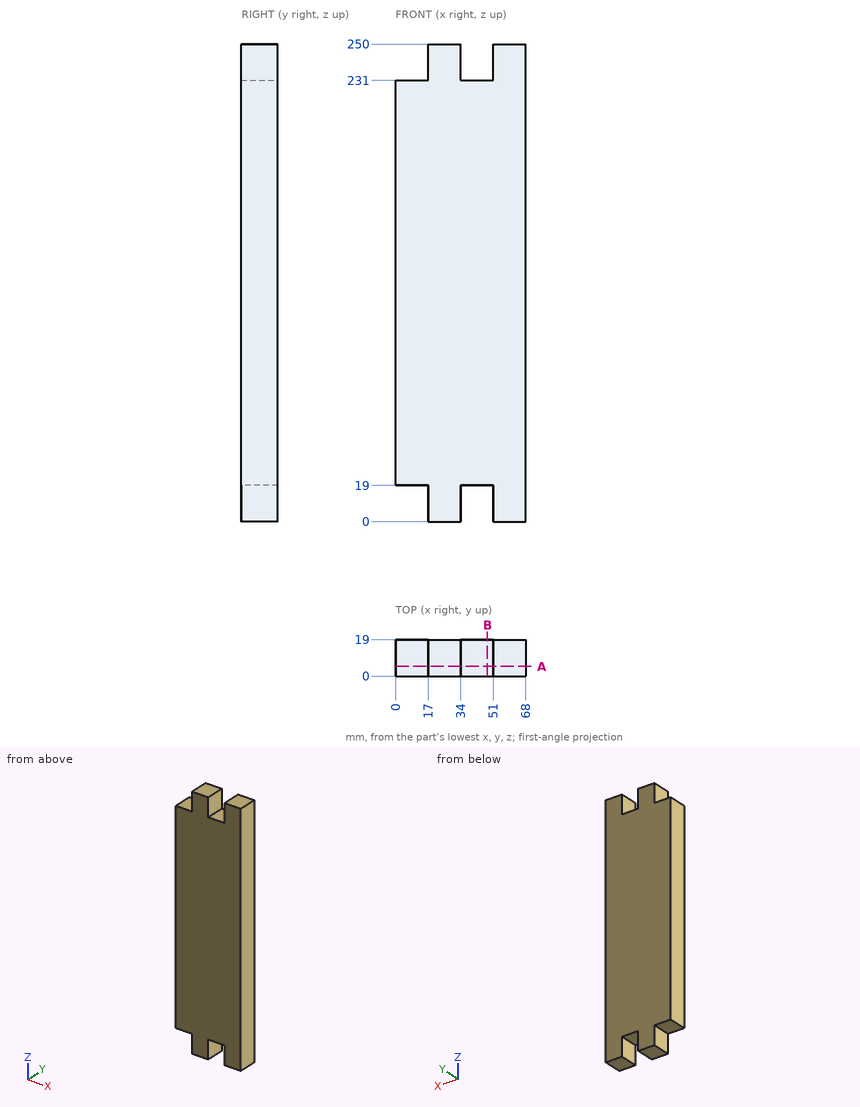
Here's the drawing with two shaded views (mm, measured from the low corner). I have some questions. Give positions to 0.01 mm unless a question says otherwise; leave off trailing zeros. Write each loop counter-clockwise with the first axis right and the second up, starting at its lowest first coordinate (ties: lowest second). Pieces come first, ordered by that corner, then holes. Notation, with made-up numbers: (-37.75, 1) -> (-2.75, 1) arc R23 cw to (-2.75, 29) -> close; hole circle Ø11 at (47, 31). An arc over 180 degrees is marked (long way). Use one line per item in the form item = value.
1) If I drill on L1, parallel to Z at x = 7.5, y = 6.5, over which ranges is the centre line in solid material (lowest first)? Write a range as [from, to].
Verdict:
L1 = [19, 231]
2) I'm going to push flat-ended pins straight in: pin 1 (9.5 mm diameter, centred on y = 12, z = 236, fed in from -X); pin 2 (8.5 mm diameter, centred on x = 4.5, y = 14, fed in from -Z); pin 3 (5 mm diameter, centred on x = 44.5, y = 2.5, fed in from +Z). Where does each tip first touch, or does it pass through?
Verdict:
pin_1 = 17
pin_2 = 19
pin_3 = 231
3) Suppose I cut it at A-A (y = 5). Please give me the cut outline in (x, z).
Verdict:
outline = (0, 19) -> (17, 19) -> (17, 0) -> (34, 0) -> (34, 19) -> (51, 19) -> (51, 0) -> (68, 0) -> (68, 250) -> (51, 250) -> (51, 231) -> (34, 231) -> (34, 250) -> (17, 250) -> (17, 231) -> (0, 231) -> close
4) Suppose I cut it at B-B (x = 48). Please give me the cut outline in (y, z).
Verdict:
outline = (0, 19) -> (19, 19) -> (19, 231) -> (0, 231) -> close
